Input: part model. Units: mm. Frame: model coordinates. A direction names the side the tool comes from. Give positions to 0.01 mm unless a question says otherwise; leave off trailing zeros. Order: outer loops, then holes, each group sorted by start corner. A loop starts at its lowest first (then second) coordinate and runs counter-clockwise, first axis right, second up. Notation, with made-up numbers: (63.25, 59) - (88.25, 59) arc R12 ccw to (88.25, 69) - close; hole circle Ø11 at (7.25, 48). An arc over 180 degrees is marked (long way). Use a Markdown table: item, result.
Autodesk Inventor part; units mm, degrees
ref_plane "bolt_XY" through (-3.4, 0, 0) normal (1, 0, 0) x (0, 0, -1)
ref_plane "bolt_YZ" through (-3.4, 0, 0) normal (0, 0, -1) x (0, 1, 0)
ref_plane "bolt_ZX" through (-3.4, 0, 0) normal (0, 1, 0) x (1, 0, 0)
sketch "Sketch_1" plane through (0, 0, 0) normal (0, 0, 1) x (1, 0, 0)
  line L0 (4.6, 0) -> (-3.4, 0)
  line L1 (-3.4, 0) -> (-3.4, 6)
  line L2 (-3.4, 6) -> (-3, 6)
  line L3 (-3, 6) -> (0.131, 2.869)
  arc A0 (0.131, 2.869) -> (0.5553, 2.6932) centre (0.5553, 3.2932) ccw
  line L4 (0.5553, 2.6932) -> (1, 2.6932)
  line L5 (1, 2.6932) -> (2, 3)
  line L6 (2, 3) -> (4.6, 3)
  line L7 (4.6, 3) -> (4.6, 0)
  line L8 (4.6, 0) -> (-3.4, 0)
revolve "Revolution1" add sketch "Sketch_1" angle 360 about axis through (4.6, 0, 0) along (1, 0, 0)
thread "Thread1"
sketch "Sketch_2" plane through (-3.4, 0, 0) normal (1, 0, 0) x (0, 0, -1)
  line L0 (-3.35, -0.8) -> (-2, -0.8)
  arc A0 (-0.8, -2) -> (-2, -0.8) centre (-2, -2) ccw
  line L1 (-0.8, -2) -> (-0.8, -3.35)
  line L2 (-0.8, -3.35) -> (0.8, -3.35)
  line L3 (0.8, -3.35) -> (0.8, -2)
  arc A1 (2, -0.8) -> (0.8, -2) centre (2, -2) ccw
  line L4 (2, -0.8) -> (3.35, -0.8)
  line L5 (3.35, -0.8) -> (3.35, 0.8)
  line L6 (3.35, 0.8) -> (2, 0.8)
  arc A2 (0.8, 2) -> (2, 0.8) centre (2, 2) ccw
  line L7 (0.8, 2) -> (0.8, 3.35)
  line L8 (0.8, 3.35) -> (-0.8, 3.35)
  line L9 (-0.8, 3.35) -> (-0.8, 2)
  arc A3 (-2, 0.8) -> (-0.8, 2) centre (-2, 2) ccw
  line L10 (-2, 0.8) -> (-3.35, 0.8)
  line L11 (-3.35, 0.8) -> (-3.35, -0.8)
extrude "Extrusion1" cut sketch "Sketch_2" along normal blind 1.7
ref_plane "bolt_XY" through (-3.4, 0, 0) normal (1, 0, 0) x (0, 0, -1)
ref_plane "bolt_YZ" through (-3.4, 0, 0) normal (0, 0, -1) x (0, 1, 0)
ref_plane "bolt_ZX" through (-3.4, 0, 0) normal (0, 1, 0) x (1, 0, 0)
ref_plane "nut_XY" through (4.6, 0, 0) normal (1, 0, 0) x (0, 0, -1)
ref_plane "nut_YZ" through (4.6, 0, 0) normal (0, 0, -1) x (0, 1, 0)
ref_plane "nut_ZX" through (4.6, 0, 0) normal (0, 1, 0) x (1, 0, 0)
properties part number "SFBJ6-8"
1. Section query A-A (y = 0). Return loops of the section in (x, z).
Response:
| item | result |
|---|---|
| outline | (-3.4, -6) - (-3, -6) - (0.13, -2.87) arc R0.6 cw to (0.56, -2.69) - (1, -2.69) - (2, -3) - (4.6, -3) - (4.6, 3) - (2, 3) - (1, 2.69) - (0.56, 2.69) arc R0.6 cw to (0.13, 2.87) - (-3, 6) - (-3.4, 6) - (-3.4, 3.35) - (-1.7, 3.35) - (-1.7, -3.35) - (-3.4, -3.35) - close |
2. Section query C-C (x = 2.25). Return loops of the section in (y, z).
Response:
| item | result |
|---|---|
| outline | circle Ø6 at (0, 0) |
3. Set-up query: faces 1 (the face through (-3, 0, 3.35)), 2 (the face through (0.78, -2.69, 0.12)), 3 (the face through (4.6, 0, 0)). Return all of +Z, -Z, +X, -X, +Y, -Y with unobstructed straight access to the full face (end or side cutting, diameter ignored); none if empty.
Response:
| item | result |
|---|---|
| face 1 | -X |
| face 2 | none |
| face 3 | +Z, -Z, +X, +Y, -Y |
4. Mould query, pull axis Z, two halves, no side actions, for faces 4 (the face through (-3.4, 1.2, 1.4)), 5 (the face through (-3, 3.35, 0)), 6 (the face through (3, -3, 0)). Classes: pulls with the +Z half, pulls with the -Z half, needs draft (parallel to the pull), parting line crosses it, or undercut.
Response:
| item | result |
|---|---|
| face 4 | needs draft |
| face 5 | undercut |
| face 6 | parting line crosses it |
5. Material intervals for line 1 along Y through (x, z) = (-2.25, 1.5); line 2 along Z through (x, y) = (-2.25, 2.75); line 3 along Y through (x, z) = (-2.25, 0.25), sorted ascending.
Response:
| item | result |
|---|---|
| line 1 | y = -5.03 to -0.91, 0.91 to 5.03 |
| line 2 | z = -4.47 to -0.8, 0.8 to 4.47 |
| line 3 | y = -5.24 to -3.35, 3.35 to 5.24 |
6. Pin query (flat end, axial travel): pin 1 (0.7 mm diameter, centred on x = -3, z = -3, fed in from +Y); pin 2 (1.3 mm diameter, centred on x = -2.5, z = -0.5, fed in from +Y); pin 3 (1.1 mm diameter, centred on x = -2.5, y = 3, fed in from +Z); pin 4 (0.8 mm diameter, centred on x = -2.5, z = 0, fed in from -Y). Return the tip coordinate at first contact, or that it passes through.
Response:
| item | result |
|---|---|
| pin 1 | stops at y = 5.38 |
| pin 2 | stops at y = 6 |
| pin 3 | stops at z = 5.32 |
| pin 4 | stops at y = -5.9 |
